For this review, take the finished solid that the model builds, in its own axes (mm). A direction names the side the tool comes from. Give positions to 0.01 mm unless a question says otherwise; leave off trailing zeros. Order: outer loops, then holes, each group sorted by start corner. A loop starts at its lowest first (then second) coordinate and runs counter-clockwise, first axis right, second up. Notation, with made-up numbers: (11.5, -25.75) -> (62.5, -25.75) arc R18 ccw to (62.5, 8.25) -> close; hole circle Ø1 at (51.25, -4.75). An arc over 180 degrees is marked (long way). Use CSV: the item, a comma, the result in double quotes. Start each with the question number.
```python
from build123d import *

# Parameters (mm, degrees)
SKETCH_2_W          = 4.5
SKETCH_2_H          = 28
CUT_EXTRUDE_1_DEPTH = 10
SKETCH_3_R          = 4.25
CUT_EXTRUDE_2_DEPTH = 20


with BuildPart() as part:
    # ｽｹｯﾁ1 → 回転1 (revolve)
    with BuildSketch(Plane.XY, mode=Mode.PRIVATE) as revolve_1_sk:
        Polygon((-78, 0), (-78, 12.5), (-73, 12.5), (-73, 15), (-50, 15), (-50, 12.5), (-1, 12.5), (0, 11.5), (0, 0), align=None)
    revolve(revolve_1_sk.sketch.rotate(Axis((-78, 0, 0), (1, 0, 0)), 90), axis=Axis((-78, 0, 0), (1, 0, 0)))

    # ｽｹｯﾁ2 → ｶｯﾄ - 押し出し1 (cut)
    with BuildSketch(Plane(origin=(0, 0, 0), x_dir=(0, 0, -1), z_dir=(1, 0, 0))):
        with Locations((11.75, 0)):
            Rectangle(SKETCH_2_W, SKETCH_2_H)
        with Locations((-11.75, 0)):
            Rectangle(SKETCH_2_W, SKETCH_2_H)
    extrude(amount=-CUT_EXTRUDE_1_DEPTH, mode=Mode.SUBTRACT)

    # ｽｹｯﾁ3 → ｶｯﾄ - 押し出し2 (cut)
    with BuildSketch(Plane(origin=(0, 0, 0), x_dir=(0, 0, -1), z_dir=(1, 0, 0))):
        Circle(SKETCH_3_R)
    extrude(amount=-CUT_EXTRUDE_2_DEPTH, mode=Mode.SUBTRACT)


solid = part.part
```
1. Consider section B-B (z = 0). State the section outline as (x, y) points, plus the area to 3 significant figures.
2. Clearance check with flat-ended pins moving along their axes: P1, Ø5, axis at x = -31.5, y = 12, coming from the +Z side; P2, Ø10, axis at y = 6, z = -8, coming from the +X side; P3, Ø1, axis at x = -67.5, y = 3.5, coming from the -Z side; P4, Ø3, axis at x = -22.5, z = 6.5, coming from the +Y side. State where each tip first meets the part, or that it passes through.
3. For faces 1 (the face through (-5, 0, -9.5)), 2 (the face through (-75.465, -3.755, 11.923)), 3 (the face through (-25.157, -12.394, -1.627)), list the 3-axis set-ups (+Z, -Z, +X, -X, +Y, -Y) from which the entire face can be reached by the end or side of a thin tool; tool diameter is ignored.
4. Draft analysis for pull direction Z (two halves, no side actions). For faces 4 (the face through (-50, -12.3, -3.4)), 5 (the face through (-9.86, 3.584, -2.285)), 6 (the face through (-61.34, -12.65, 8.06)), state which applies: +Z half, -Z half, draft (parallel to the pull), parting line (faces both ways), or undercut.
5. Consider section C-C (x = -9). State the section outline as (y, z) points, plus the area to 3 significant figures.
6. Consider section D-D (x = -39). State the section outline as (y, z) points.
7. Consider section A-A (y = 0). State the section outline as (x, z) points.
8. To check wall thickness, follow L1, parallel to Y at x = -5, z = 0; L2, parallel to X at y = 3.5, z = 10; L3, parallel to X at y = -2, z = 3.25. State the ranges of each line that lie inside material, in increasing order. Write a range as [from, to].
Answer list:
1,outline,"(-78, -12.5) -> (-73, -12.5) -> (-73, -15) -> (-50, -15) -> (-50, -12.5) -> (-1, -12.5) -> (0, -11.5) -> (0, -4.25) -> (-20, -4.25) -> (-20, 4.25) -> (0, 4.25) -> (0, 11.5) -> (-1, 12.5) -> (-50, 12.5) -> (-50, 15) -> (-73, 15) -> (-73, 12.5) -> (-78, 12.5) -> close"
1,area,"1,890 mm2"
2,P1,"z = 8.12"
2,P2,"x = 0"
2,P3,"z = -14.7"
2,P4,"y = 11.46"
3,face 1,"-Z, +X, +Y, -Y"
3,face 2,"-X"
3,face 3,"+X"
4,face 4,"draft"
4,face 5,"undercut"
4,face 6,"parting line"
5,outline,"(-8.12, -9.5) -> (8.12, -9.5) arc R12.5 ccw to (8.12, 9.5) -> (-8.12, 9.5) arc R12.5 ccw to start; hole circle Ø8.5 at (0, 0)"
5,area,"367 mm2"
6,outline,"circle Ø25 at (0, 0)"
7,outline,"(-78, -12.5) -> (-73, -12.5) -> (-73, -15) -> (-50, -15) -> (-50, -12.5) -> (-10, -12.5) -> (-10, -9.5) -> (0, -9.5) -> (0, -4.25) -> (-20, -4.25) -> (-20, 4.25) -> (0, 4.25) -> (0, 9.5) -> (-10, 9.5) -> (-10, 12.5) -> (-50, 12.5) -> (-50, 15) -> (-73, 15) -> (-73, 12.5) -> (-78, 12.5) -> close"
8,L1,"[-12.5, -4.25], [4.25, 12.5]"
8,L2,"[-78, -10]"
8,L3,"[-78, -20]"
